```python
from build123d import *

# Parameters (mm, degrees)
F0_R     = 2.5
F1_DEPTH = 1
F2_R     = 1.85
F3_DEPTH = 1
F4_R     = 2.5
F4_R_2   = 1.85
F5_DEPTH = 43
F6_R     = 1.85
F7_DEPTH = 1
F8_R     = 2.5
F8_R_2   = 1.85
F9_DEPTH = 1
F10_SIZE = 0.5


with BuildPart() as f1:
    # F0 (on Front) → F1 (new body)
    with BuildSketch(Plane.XZ):
        Circle(F0_R)
    extrude(amount=F1_DEPTH)

    # F2 (on face) → F3 (join)
    with BuildSketch(Plane.XZ.offset(1)):
        Circle(F2_R)
    extrude(amount=F3_DEPTH)

    # F4 (on face) → F5 (join)
    with BuildSketch(Plane.XZ.offset(2)):
        Circle(F4_R)
        Circle(F4_R_2, mode=Mode.SUBTRACT)
        Circle(F4_R_2)
    extrude(amount=F5_DEPTH)

    # F6 (on face) → F7 (join)
    with BuildSketch(Plane.XZ.offset(45)):
        Circle(F6_R)
    extrude(amount=F7_DEPTH)

    # F8 (on face) → F9 (join)
    with BuildSketch(Plane.XZ.offset(46)):
        Circle(F8_R)
        Circle(F8_R_2, mode=Mode.SUBTRACT)
        Circle(F8_R_2)
    extrude(amount=F9_DEPTH)

    # F10
    f10_edges = [f1.edges().sort_by_distance(p)[0] for p in [
        (-2.5, -47, 0),
        (-2.5, 0, 0),
    ]]
    chamfer(f10_edges, length=F10_SIZE)


solid = f1.part
```
Verification items for the finished model (mm, model axes). A direction names the side the tool comes from. Coordinates: 2 decimals unless noted, no trailing zeros. Loops run counter-clockwise (first coordinate to the right, second up) from the corner with the lowest first, then second, coordinate; pieces in that order, holes last. Notation, with made-up numbers: (-23.5, 34.5) - (34.5, 34.5) arc R23 ccw to (34.5, 62.5) - close; hole circle Ø7 at (-20.5, -3.5). An arc over 180 degrees is marked (long way). Put each result on its own line as item: value.
Item 1: Draft check along Y on faces 3 (the face through (-0.54, -46.25, -2.44)), 4 (the face through (-2, -45, 1)), 5 (the face through (0, -47, 0)). Enter one of: pulls with the +Y half, pulls with the -Y half, needs draft (parallel to the pull), parting line crosses it, or undercut.
Conclusion:
face 3: needs draft
face 4: undercut
face 5: pulls with the -Y half
Item 2: Scan lines: line 1 along Y through (x, z) = (1.05, -2); line 2 along Y through (x, z) = (1.05, 1.9); line 3 along Z through (x, y) = (1.5, -13). Record each from-to range of solid material in increasing order.
Conclusion:
line 1: y = -46.74 to -46, -45 to -2, -1 to -0.26
line 2: y = -46.83 to -46, -45 to -2, -1 to -0.17
line 3: z = -2 to 2
Item 3: Section check A-A (y = -15). Enter the section's corners in (x, z), then the cut area to 3 significant figures.
Conclusion:
outline: circle Ø5 at (0, 0)
area: 19.6 mm2
Item 4: Set-up check for faces 1 (the face through (-2, -46, 1)), 2 (the face through (0, 0, 0)): record each of +Z, -Z, +X, -X, +Y, -Y from which the full face is reachable in a straight line by a thin tool's end or side.
Conclusion:
face 1: none
face 2: +Z, -Z, +X, -X, +Y
